Read the model definition and answer for the solid it produces. Units are mm, in the model's axes. Face numbers are marked on the shaded views. A direction names the side the tool comes from. Round coordinates to 2 decimals unless told otherwise and drop trailing zeros. Write each loop counter-clockwise with the first axis right and the second up, starting at its lowest first coordinate (ties: lowest second). Pieces come first, ordered by that corner, then holes. Notation, with made-up numbers: (43.25, 57.5) - (79.25, 57.5) arc R19 cw to (79.25, 92.5) - close; hole circle Ø10 at (-23, 81.25). An arc over 180 degrees is marked (long way). One line per item, written item: value. Start each with the question number.
(1) A cutting plane is placed at B-B, the plane x = 41. Determine the outline of the cut face in (y, z).
(2) A cutting plane is placed at A-A, the plane y = 10.5. Determine the outline of the cut face in (x, z).
(3) For the marked faces 1 and 2, determine the directions among +Z, -Z, +X, -X, +Y, -Y from which every point of the face is accessible in a straight line to the end or side of a thin tool.
(4) Flat-ended cylindrical pins translate along their axes: pin 1 Ø0.8 at (y, z) = (10.5, -1.5) entering from +X; pin 2 Ø0.5 at (y, z) = (24, -1.5) entering from -X; pin 3 Ø1 at (x, z) = (28.5, -2) entering from +Y. Find the tip coordinate at first contact, or state that the pin passes through.
(5) Find the intervals of material crossed by L1, parallel to Y at x = 36, z = -1.85; L2, parallel to X at y = 33, z = -1.4; L3, parallel to X at y = 17, z = -1.25, in increasing order.
from build123d import *

# Parameters (mm, degrees)
SKETCH_1_W      = 52
SKETCH_1_H      = 41
SKETCH_1_W_2    = 46
SKETCH_1_H_2    = 35
EXTRUDE_1_DEPTH = 1
SKETCH_1_3_W    = 46
SKETCH_1_3_H    = 35
SKETCH_1_3_W_2  = 36.5
SKETCH_1_3_H_2  = 29
EXTRUDE_2_DEPTH = 2
FILLET_2_R      = 2
CHAMFER_1_SIZE  = 1.6


with BuildPart() as part:
    # Эскиз1 → Бобышка-Вытянуть1 (new body)
    with BuildSketch(Plane.XY):
        with Locations((23, 17.5)):
            Rectangle(SKETCH_1_W, SKETCH_1_H)
        with Locations((23, 17.5)):
            Rectangle(SKETCH_1_W_2, SKETCH_1_H_2, mode=Mode.SUBTRACT)
    extrude(amount=-EXTRUDE_1_DEPTH)

    # Эскиз1<3> → Бобышка-Вытянуть2 (add)
    with BuildSketch(Plane.XY):
        with Locations((23, 17.5)):
            Rectangle(SKETCH_1_3_W, SKETCH_1_3_H)
        with Locations((26.25, 17)):
            Rectangle(SKETCH_1_3_W_2, SKETCH_1_3_H_2, mode=Mode.SUBTRACT)
    extrude(amount=-EXTRUDE_2_DEPTH)

    # Скругление2
    fillet_2_edges = [part.edges().sort_by_distance(p)[0] for p in [
        (-3, -3, -0.5),
        (-3, 38, -0.5),
        (49, 38, -0.5),
        (49, -3, -0.5),
        (46, 0, -1.5),
        (0, 0, -1.5),
        (0, 35, -1.5),
        (46, 35, -1.5),
    ]]
    fillet(fillet_2_edges, radius=FILLET_2_R)

    # Фаска1
    chamfer_1_edges = [part.edges().sort_by_distance(p)[0] for p in [
        (44.5, 17, 0),
        (26.25, 2.5, 0),
        (8, 17, 0),
        (26.25, 31.5, 0),
    ]]
    chamfer(chamfer_1_edges, length=CHAMFER_1_SIZE)


solid = part.part
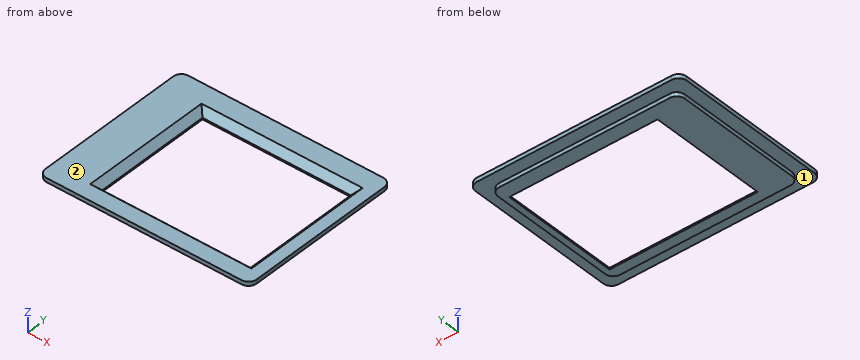
Here are the results:
1. outline: (-3, -1) - (0, -1) - (0, -2) - (2.5, -2) - (2.5, -1.6) - (0.9, 0) - (-3, 0) - close; (31.5, -2) - (35, -2) - (35, -1) - (38, -1) - (38, 0) - (33.1, 0) - (31.5, -1.6) - close
2. outline: (-3, -1) - (0, -1) - (0, -2) - (8, -2) - (8, -1.6) - (6.4, 0) - (-3, 0) - close; (44.5, -2) - (46, -2) - (46, -1) - (49, -1) - (49, 0) - (46.1, 0) - (44.5, -1.6) - close
3. face 1: -Z
3. face 2: +Z, +X, -X, +Y, -Y
4. pin 1: x = 46
4. pin 2: x = 0
4. pin 3: y = 35
5. L1: 0 to 2.5, 31.5 to 35
5. L2: 0 to 46
5. L3: 0 to 7.65, 44.85 to 46
